```python
from build123d import *

# Parameters (mm, degrees)
SKETCH1_R           = 1.7145
BOSS_EXTRUDE1_DEPTH = 4.572
CUT_EXTRUDE1_DEPTH  = 3.81
CUT_EXTRUDE2_DEPTH  = 111.125


with BuildPart() as part:
    # Sketch1 → Boss-Extrude1 (new body)
    with BuildSketch(Plane(origin=(0, 0, 0), x_dir=(1, 0, 0), z_dir=(0, 1, 0))):
        Polygon((-4.445, 0), (0, 0), (0, 20.32), (-38.1, 20.32), (-38.1, 127), (-62.484, 127), (-62.484, 20.32), (-100.584, 20.32), (-100.584, 0), (-62.484, 0), (-62.484, -9.525), (-38.1, -9.525), (-38.1, 0), align=None)
        with Locations(Location((-96.139, 5.969, 0), (0, 0, 270))):
            Circle(SKETCH1_R, mode=Mode.SUBTRACT)
        with Locations(Location((-70.739, 5.969, 0), (0, 0, 270))):
            Circle(SKETCH1_R, mode=Mode.SUBTRACT)
        with Locations(Location((-29.845, 5.969, 0), (0, 0, 270))):
            Circle(SKETCH1_R, mode=Mode.SUBTRACT)
        with Locations(Location((-4.445, 5.969, 0), (0, 0, 270))):
            Circle(SKETCH1_R, mode=Mode.SUBTRACT)
        with Locations(Location((-50.292, 120.0404, 0), (0, 0, 270))):
            Circle(SKETCH1_R, mode=Mode.SUBTRACT)
    extrude(amount=BOSS_EXTRUDE1_DEPTH)

    # Sketch2 → Cut-Extrude1 (cut)
    with BuildSketch(Plane.XY.offset(9.525)):
        with BuildLine():
            Line((-53.086, 4.572), (-47.498, 4.572))
            ThreePointArc((-47.498, 4.572), (-50.292, 1.778), (-53.086, 4.572))
        make_face()
    extrude(amount=-CUT_EXTRUDE1_DEPTH, mode=Mode.SUBTRACT)

    # Sketch3 → Cut-Extrude2 (cut)
    with BuildSketch(Plane.XY.offset(5.715)):
        with BuildLine():
            Line((-53.5432, 4.572), (-47.0408, 4.572))
            ThreePointArc((-47.0408, 4.572), (-50.292, 1.3208), (-53.5432, 4.572))
        make_face()
    extrude(amount=-CUT_EXTRUDE2_DEPTH, mode=Mode.SUBTRACT)


solid = part.part
```
The listing builds one solid part. Answer for the finished solid, in the listing's coordinates (mm). A direction names the side the tool comes from. Give positions to 0.01 mm unless a question says otherwise; leave off trailing zeros. Order: outer loops, then holes, each group sorted by start corner. A loop starts at its lowest first (then second) coordinate and runs counter-clockwise, first axis right, second up.
1) For faces 4 (the face through (-62.484, 2, 5)), 5 (the face through (-19, 2, -20.32)), 6 (the face through (-62.484, 2, -74)), 7 (the face through (-50.23, 1.78, 7.65)), determine the directions among +Z, -Z, +X, -X, +Y, -Y from which every point of the face is accessible in a straight line to the end or side of a thin tool.
Reported:
face 4: +Z, -X, +Y, -Y
face 5: -Z, +X, +Y, -Y
face 6: -Z, -X, +Y, -Y
face 7: +Z, +Y
2) Given P1, Ø2.5, axis at x = -11.5, y = 2.5, coming from the +Z side; P2, Ø2.5, axis at y = 3.5, z = -52.5, coming from the -X side; P3, Ø1.6, axis at x = -50, y = 3.5, coming from the +Z side, each flat-ended and moving along its own axis, determine where each tip first touches the part or whether it passes through.
Reported:
P1: stops at z = 0
P2: stops at x = -62.48
P3: stops at z = -105.41
3) Find section D-D on z = -16.5. Write down the section's boundary in (x, y).
Reported:
outline: (-100.58, 0) - (0, 0) - (0, 4.57) - (-47.04, 4.57) arc R3.25 cw to (-53.54, 4.57) - (-100.58, 4.57) - close
4) Find section B-B on z = -84. Write down the section's boundary in (x, y), then the cut area to 3 significant figures.
Reported:
outline: (-62.48, 0) - (-38.1, 0) - (-38.1, 4.57) - (-47.04, 4.57) arc R3.25 cw to (-53.54, 4.57) - (-62.48, 4.57) - close
area: 94.9 mm2
5) Determine the mould class of faces 1 (the face through (-19, 2, 0)), 2 (the face through (-81, 2, -20.32)), 3 (the face through (-31.52, 2.25, -6.34)) for opening direction Z: pulls with the +Z half, pulls with the -Z half, needs draft (parallel to the pull), parting line crosses it, or undercut.
Reported:
face 1: pulls with the +Z half
face 2: pulls with the -Z half
face 3: undercut
6) Consider line 1 along Z through (x, y) = (-50, 1.55) (3 decimals); line 2 along Z through (x, y) = (-50, 0.7) (3 decimals); line 3 along Z through (x, y) = (-32, 0.25). Determine where each line is inside the solid, lowest interval first.
Reported:
line 1: z = -127 to -121.73, -118.351 to -105.41, 5.715 to 9.525
line 2: z = -127 to -121.73, -118.351 to 9.525
line 3: z = -20.32 to 0
7) Find section C-C on x = -83.5. Write down the section's boundary in (y, z).
Reported:
outline: (0, -20.32) - (4.57, -20.32) - (4.57, 0) - (0, 0) - close
8) Find section A-A on y = 3.15. Write down the section's boundary in (x, z) (1 decimal), then the cut area to 3 significant figures.
Reported:
outline: (-100.6, -20.3) - (-62.5, -20.3) - (-62.5, -127) - (-38.1, -127) - (-38.1, -20.3) - (0, -20.3) - (0, 0) - (-38.1, 0) - (-38.1, 9.5) - (-47.9, 9.5) - (-47.9, 5.7) - (-47.4, 5.7) - (-47.4, -105.4) - (-53.2, -105.4) - (-53.2, 5.7) - (-52.7, 5.7) - (-52.7, 9.5) - (-62.5, 9.5) - (-62.5, 0) - (-100.6, 0) - close; hole circle Ø3.4 at (-96.1, -6); hole circle Ø3.4 at (-70.7, -6); hole circle Ø3.4 at (-50.3, -120); hole circle Ø3.4 at (-29.8, -6); hole circle Ø3.4 at (-4.4, -6)
area: 4,160 mm2
